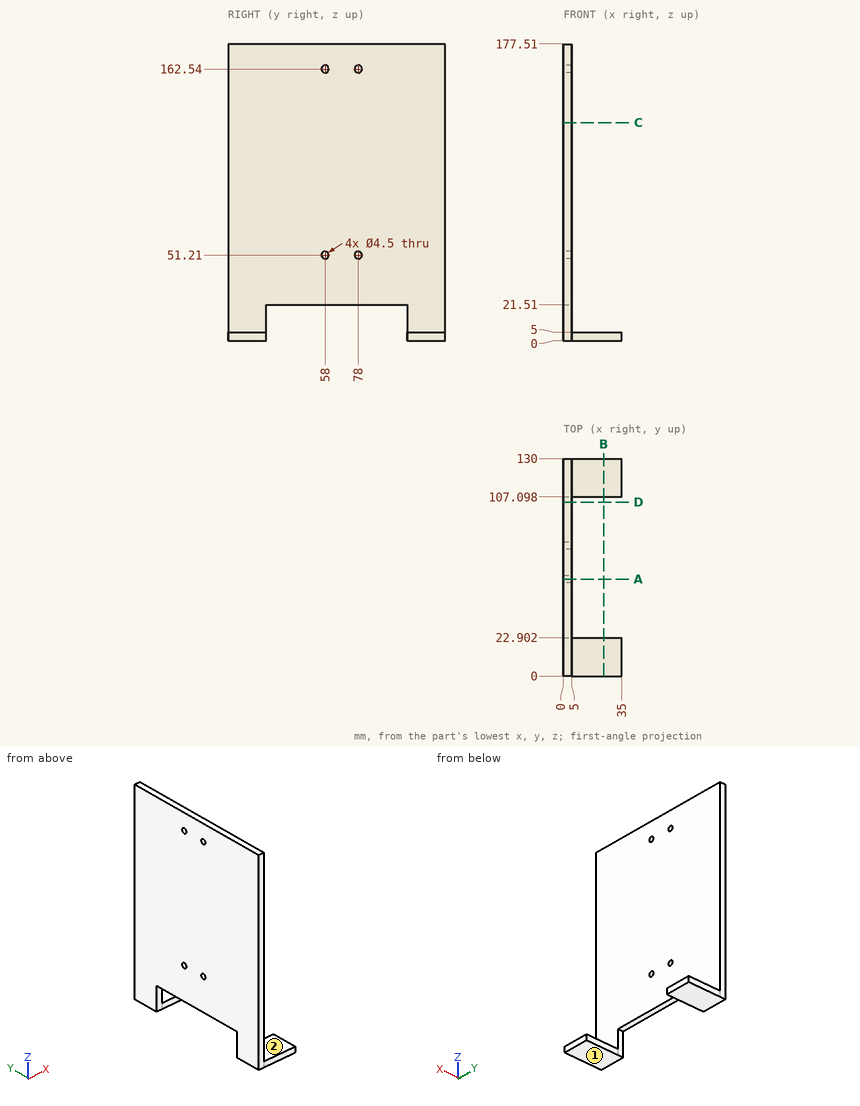
Drawing for the job (mm, zero at the part's lowest x, y, z). A direction names the side the tool comes from. Round coordinates to 2 decimals unless told otherwise and drop trailing zeros. Write each loop counter-clockwise with the first axis right and the second up, starting at its lowest first coordinate (ties: lowest second). Pieces come first, ordered by that corner, then holes. Notation, with made-up numbers: M -17.75,73.25 L 27.25,73.25 A20 ccw 27.25,88.25 Z; hole C 33,9 d10. An arc over 180 degrees is marked long. One line per question, with ' | ' between items.
1. Cut at D-D on y = 104. Write the cut outline in (x, z), and give its area (3 significant figures).
Working result:
outline: M 0,21.51 L 5,21.51 L 5,177.51 L 0,177.51 Z | area: 780 mm2
2. Cut at B-B on x = 24. Write the cut outline in (y, z).
Working result:
outline: M 0,0 L 22.9,0 L 22.9,5 L 0,5 Z; M 107.1,0 L 130,0 L 130,5 L 107.1,5 Z
3. Which spindle directions (+Z, -Z, +X, -X, +Y, -Y) get a long thin tool onto all of the face, cutting with end or side? Do the marked faces 1 and 2. Say none if no direction does.
Working result:
face 1: -Z, +X, -X, +Y, -Y | face 2: +Z, +X, +Y, -Y
4. Cut at A-A on y = 58. Write the cut outline in (x, z).
Working result:
outline: M 0,21.51 L 5,21.51 L 5,48.96 L 0,48.96 Z; M 0,53.46 L 5,53.46 L 5,160.29 L 0,160.29 Z; M 0,164.79 L 5,164.79 L 5,177.51 L 0,177.51 Z
5. Pin check, flat tips, straight feed: pin 1 Ø4 at (y, z) = (78, 51.21) entering from +X; pin 2 Ø18.5 at (x, y) = (22.5, 118.5) entering from +Z; pin 3 Ø5.5 at (x, y) = (1.5, 54.5) entering from -Z; pin 4 Ø6 at (y, z) = (78, 162.54) entering from +X. Stop position of each tip, or through.
Working result:
pin 1: through | pin 2: z = 5 | pin 3: z = 21.51 | pin 4: x = 5
6. Cut at C-C on z = 130.5. Write the cut outline in (x, y), and give its area (3 significant figures).
Working result:
outline: M 0,0 L 5,0 L 5,130 L 0,130 Z | area: 650 mm2
7. Probe L1, parallel to Z at x = 1.25, y = 58; L2, parallel to X at y = 84, z = 102.5. List the from-to ranges inside material, lowest first. Write a range as from..to.
Working result:
L1: 21.51..48.96, 53.46..160.29, 164.79..177.51 | L2: 0..5
